```python
from build123d import *

# Parameters (mm, degrees)
F0_W     = 600
F0_H     = 500
F1_DEPTH = 20
F2_W     = 20
F2_H     = 20
F3_DEPTH = 20
F4_W     = 580
F4_H     = 10
F5_DEPTH = 10


with BuildPart() as f1:
    # F0 (on Front) → F1 (new body)
    with BuildSketch(Plane.XZ):
        Rectangle(F0_W, F0_H)
    extrude(amount=F1_DEPTH)

    # F2 (on face) → F3 (cut, through all)
    with BuildSketch(Plane.XZ.offset(20)):
        with Locations((290, -220)):
            Rectangle(F2_W, F2_H)
        with Locations((290, -180)):
            Rectangle(F2_W, F2_H)
        with Locations((290, -140)):
            Rectangle(F2_W, F2_H)
        with Locations((290, -100)):
            Rectangle(F2_W, F2_H)
        with Locations((290, -60)):
            Rectangle(F2_W, F2_H)
        with Locations((290, -20)):
            Rectangle(F2_W, F2_H)
        with Locations((290, 20)):
            Rectangle(F2_W, F2_H)
        with Locations((290, 60)):
            Rectangle(F2_W, F2_H)
        with Locations((290, 100)):
            Rectangle(F2_W, F2_H)
        with Locations((290, 140)):
            Rectangle(F2_W, F2_H)
        with Locations((290, 180)):
            Rectangle(F2_W, F2_H)
        with Locations((-290, -220)):
            Rectangle(F2_W, F2_H)
        with Locations((-290, -60)):
            Rectangle(F2_W, F2_H)
        with Locations((-290, 100)):
            Rectangle(F2_W, F2_H)
        with Locations((-290, 20)):
            Rectangle(F2_W, F2_H)
        with Locations((-290, 180)):
            Rectangle(F2_W, F2_H)
        with Locations((-290, -20)):
            Rectangle(F2_W, F2_H)
        with Locations((-290, 140)):
            Rectangle(F2_W, F2_H)
        with Locations((-290, 60)):
            Rectangle(F2_W, F2_H)
        with Locations((-290, -100)):
            Rectangle(F2_W, F2_H)
        with Locations((-290, -140)):
            Rectangle(F2_W, F2_H)
        with Locations((-290, -180)):
            Rectangle(F2_W, F2_H)
        with Locations((290, 220)):
            Rectangle(F2_W, F2_H)
        with Locations((-290, 220)):
            Rectangle(F2_W, F2_H)
    extrude(amount=-F3_DEPTH, mode=Mode.SUBTRACT)

    # F4 (on face) → F5 (cut)
    with BuildSketch(Plane.XZ.offset(20)):
        with Locations((0, -235)):
            Rectangle(F4_W, F4_H)
    extrude(amount=-F5_DEPTH, mode=Mode.SUBTRACT)


solid = f1.part
```
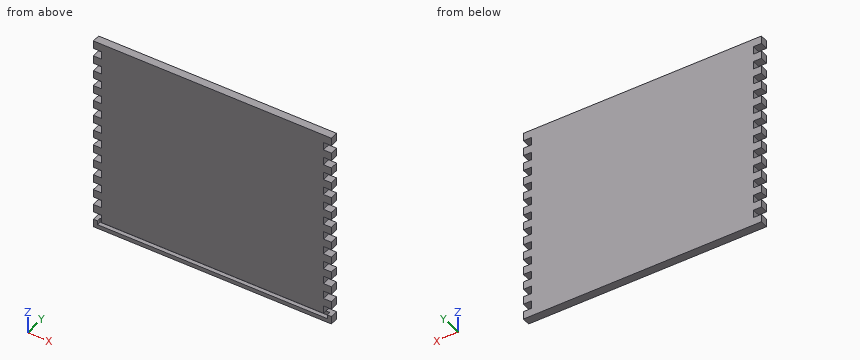
Here's how the part is built. I have some questions about the finished solid (model axes, mm). Coordinates: 2 decimals unless noted, no trailing zeros. Loops run counter-clockwise (first coordinate to the right, second up) from the corner with the lowest first, then second, coordinate; pieces in that order, holes last. Notation, with made-up numbers: M -28.5,-24 L 25.5,-24 A23 cw 25.5,-16 Z; hole C 77.5,22.25 d11. An arc over 180 degrees is marked long. One line per item, written item: value.
1. Will this pin go through, and if not, where does the flat tip stop? pin 1 Ø10 at (y, z) = (-6, -177) entering from -X.
Geometry says:
pin 1: stops at x = -280
2. Imagine slicing it at A-A (z = -217). List the corners of the cut face in (x, y) for me, and give its area (3 significant figures).
Geometry says:
outline: M -280,-20 L 280,-20 L 280,0 L -280,0 Z
area: 11,200 mm2
3. Please list where these lines run through material, in increasing order: probe 1 along Z at (x, y) = (-79, -13); probe 2 along X at (y, z) = (-15.75, 215).
Geometry says:
probe 1: z = -250 to -240, -230 to 250
probe 2: x = -280 to 280
